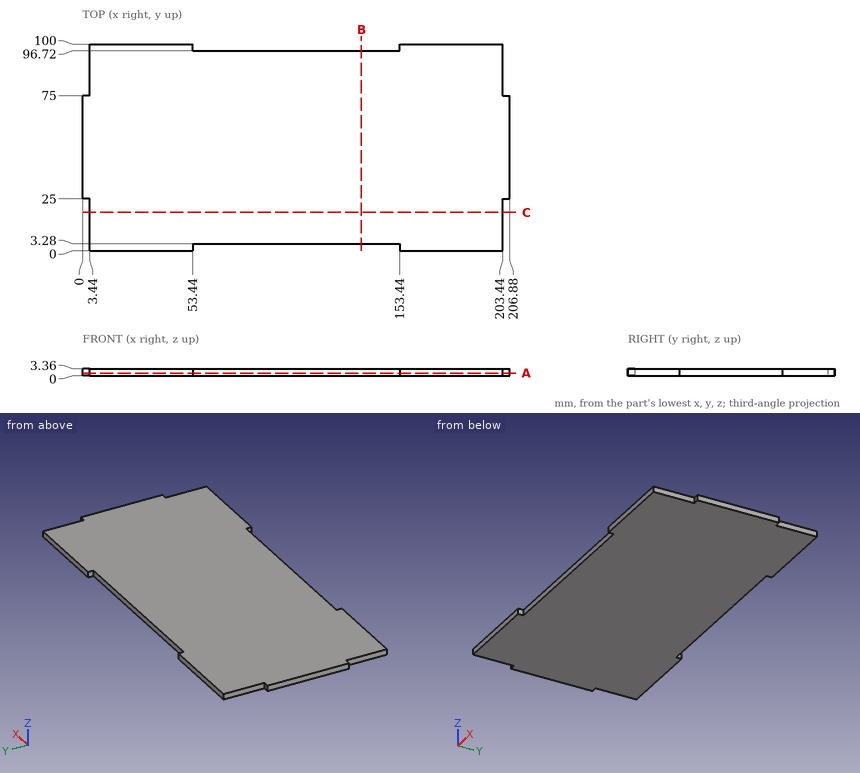
For this review, use the dimensioned drawing (mm, ordinates from the lowest corner) and the shaded views. Round coordinates to 2 decimals unless told otherwise and drop trailing zeros. Write each loop counter-clockwise with the first axis right and the second up, starting at its lowest first coordinate (ties: lowest second). Pieces come first, ordered by that corner, then holes. Notation, with made-up numbers: (60.5, 14.25) - (70.5, 14.25) arc R22 ccw to (70.5, 42.25) - close; hole circle Ø7 at (72.5, -28). An arc over 180 degrees is marked (long way). One line per item, written item: value. Start each with the question number.
1. Consider section B-B on x = 135. Write out the cut boundary in (y, z), and give its area (3 significant figures).
2. To check wall thickness, follow L1, parallel to X at y = 94, z = 1.6; L2, parallel to Y at x = 143.5, z = 2. State the ranges of each line that lie inside material, in increasing order. Write a range as from..to.
3. Clearance check with flat-ended pins moving along their axes: P1, Ø1, axis at y = 13.5, z = 1.5, coming from the +X side; P2, Ø1.6, axis at y = 98, z = 1.5, coming from the -X side; P3, Ø1.5, axis at x = 132.5, z = 1, coming from the -Y side. State where each tip first meets the part, or that it passes through.
4. Consider section C-C on y = 18.5. Write out the cut boundary in (x, z), and give its area (3 significant figures).
5. Consider section A-A on z = 1.2. Write out the cut boundary in (x, y), and give its area (3 significant figures).
Checks:
1. outline: (3.28, 0) - (96.72, 0) - (96.72, 3.36) - (3.28, 3.36) - close
1. area: 314 mm^2
2. L1: x = 3.44..203.44
2. L2: y = 3.28..96.72
3. P1: stops at x = 203.44
3. P2: stops at x = 3.44
3. P3: stops at y = 3.28
4. outline: (3.44, 0) - (203.44, 0) - (203.44, 3.36) - (3.44, 3.36) - close
4. area: 672 mm^2
5. outline: (0, 25) - (3.44, 25) - (3.44, 0) - (53.44, 0) - (53.44, 3.28) - (153.44, 3.28) - (153.44, 0) - (203.44, 0) - (203.44, 25) - (206.88, 25) - (206.88, 75) - (203.44, 75) - (203.44, 100) - (153.44, 100) - (153.44, 96.72) - (53.44, 96.72) - (53.44, 100) - (3.44, 100) - (3.44, 75) - (0, 75) - close
5. area: 19,700 mm^2
